```python
from build123d import *

# Parameters (mm, degrees)
SKETCH_1_R      = 1.5
EXTRUDE_1_DEPTH = 1.5
EXTRUDE_2_DEPTH = 15.5
SKETCH_3_W      = 49
SKETCH_3_H      = 51
EXTRUDE_3_DEPTH = 9.5
SKETCH_4_W      = 15
SKETCH_4_H      = 21
EXTRUDE_4_DEPTH = 13.5


with BuildPart() as part:
    # Эскиз1 → Бобышка-Вытянуть1 (new body)
    with BuildSketch(Plane(origin=(0, 0, 0), x_dir=(1, 0, 0), z_dir=(0, 1, 0))):
        with BuildLine():
            Line((3.5, 0), (52.5, 0))
            ThreePointArc((52.5, 0), (54.974873734, 1.025126266), (56, 3.5))
            Line((56, 3.5), (56, 83.5))
            ThreePointArc((56, 83.5), (54.974873734, 85.974873734), (52.5, 87))
            Line((52.5, 87), (3.5, 87))
            ThreePointArc((3.5, 87), (1.025126266, 85.974873734), (0, 83.5))
            Line((0, 83.5), (0, 3.5))
            ThreePointArc((0, 3.5), (1.025126266, 1.025126266), (3.5, 0))
        make_face()
        with Locations(Location((3.5, 83.5, 0), (0, 0, 270))):
            Circle(SKETCH_1_R, mode=Mode.SUBTRACT)
        with Locations(Location((52.5, 83.5, 0), (0, 0, 270))):
            Circle(SKETCH_1_R, mode=Mode.SUBTRACT)
        with Locations(Location((52.5, 25.5, 0), (0, 0, 270))):
            Circle(SKETCH_1_R, mode=Mode.SUBTRACT)
        with Locations(Location((3.5, 25.5, 0), (0, 0, 270))):
            Circle(SKETCH_1_R, mode=Mode.SUBTRACT)
    extrude(amount=EXTRUDE_1_DEPTH)

    # Эскиз2 → Бобышка-Вытянуть2 (add)
    with BuildSketch(Plane(origin=(0, 1.5, 0), x_dir=(1, 0, 0), z_dir=(0, 1, 0))):
        Polygon((20.5, 0), (28, 0), (36.5, 0), (36.5, 21), (20.5, 21), align=None)
        with BuildLine():
            Line((38.5, 21), (38.5, 0))
            Line((38.5, 0), (52.5, 0))
            ThreePointArc((52.5, 0), (53.005293538, 0.036666571), (53.5, 0.145898034))
            Line((53.5, 0.145898034), (53.5, 21))
            Line((53.5, 21), (38.5, 21))
        make_face()
    extrude(amount=EXTRUDE_2_DEPTH)

    # Эскиз3 → Бобышка-Вытянуть3 (add)
    with BuildSketch(Plane(origin=(0, 1.5, 0), x_dir=(1, 0, 0), z_dir=(0, 1, 0))):
        with Locations((28, 54.5)):
            Rectangle(SKETCH_3_W, SKETCH_3_H)
    extrude(amount=EXTRUDE_3_DEPTH)

    # Эскиз4 → Бобышка-Вытянуть4 (add)
    with BuildSketch(Plane(origin=(0, 1.5, 0), x_dir=(1, 0, 0), z_dir=(0, 1, 0))):
        with Locations((11, 10.5)):
            Rectangle(SKETCH_4_W, SKETCH_4_H)
    extrude(amount=EXTRUDE_4_DEPTH)


solid = part.part
```
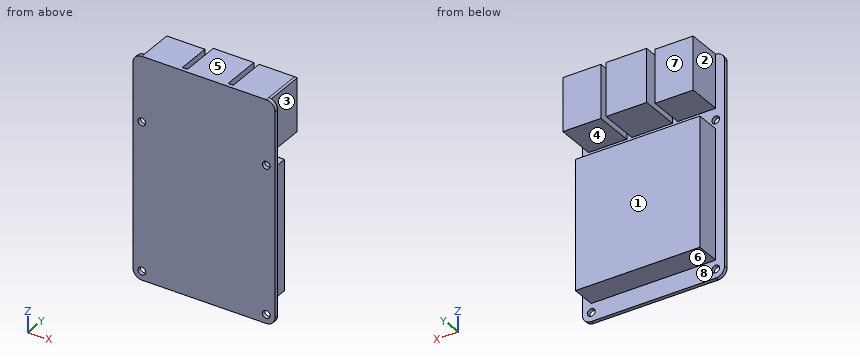
Can you work these out from the model? Positions are in its coordinate system, mm. Face numbers are marked on the shaded views. A direction names the side the tool comes from. Round coordinates to 2 decimals unless told otherwise and drop trailing zeros. Order: outer loops, then holes, each group sorted by start corner. A loop starts at its lowest first (then second) coordinate and runs counter-clockwise, first axis right, second up. Notation, with made-up numbers: (-21, 55.25) -> (1, 55.25) arc R34 cw to (1, 93.25) -> close; hole circle Ø7 at (7, 77). An arc over 180 degrees is marked (long way). Return JSON: item names as keys, results as strings. Group by question number.
1. If we section it at C-C, the plane z = -10: Write out the boundary of the cut face in (x, y), then the cut area to 3 significant figures.
2. I need wall thicknesses on line 1 (X direction, y = 0.55, z = -25.5); line 2 (X direction, y = 4, z = -16); line 3 (Z direction, x = 16, y = 9.5). Which ranges of each line are inside material? Lowest first, please. Write a range as [from, to].
3. We'd pull the mould along Z, two halves only. Please class the marked faces 6, 7 and 8: released by +Z, released by -Z, zero draft, split by the parting line, or undercut.
4. If we section it at B-B, the plane y = 9.75: Write out the boundary of the cut face in (x, z), then the cut area to 3 significant figures.
5. Will these pins go through, and if not, where does the flat tip stop? pin 1 (7 mm diameter, centred on x = 8.5, y = 5.5, fed in from -Z); pin 2 (7 mm diameter, centred on y = 11.5, z = -15.5, fed in from -X); pin 3 (1.5 mm diameter, centred on x = 21, z = -37.5, fed in from +Y); pin 4 (2.5 mm diameter, centred on x = 3.5, z = -25.5, fed in from +Y).
6. If we section it at D-D, the plane x = 9: Write out the boundary of the cut face in (y, z).
7. If we section it at A-A, the plane z = -25.5: Write out the boundary of the cut face in (x, y), then the cut area to 3 significant figures.
8. Which directions (+Z, -Z, +X, -X, +Y, -Y) give clear straight access to the entire face, cutting with the end or side of a thin tool? Please do the marked faces 1, 2, 3, 4 and 5.
Output values:
{
 "1": {"outline": "(0, 0) -> (56, 0) -> (56, 1.5) -> (53.5, 1.5) -> (53.5, 17) -> (38.5, 17) -> (38.5, 1.5) -> (36.5, 1.5) -> (36.5, 17) -> (20.5, 17) -> (20.5, 1.5) -> (18.5, 1.5) -> (18.5, 15) -> (3.5, 15) -> (3.5, 1.5) -> (0, 1.5) -> close", "area": "767 mm²"},
 "2": {"line 1": "[0, 2], [5, 51], [54, 56]", "line 2": "[3.5, 18.5], [20.5, 36.5], [38.5, 53.5]", "line 3": "[-80, -29], [-21, 0]"},
 "3": {"face 6": "released by -Z", "face 7": "zero draft", "face 8": "undercut"},
 "4": {"outline": "(3.5, -80) -> (52.5, -80) -> (52.5, -29) -> (3.5, -29) -> close; (3.5, -21) -> (18.5, -21) -> (18.5, 0) -> (3.5, 0) -> close; (20.5, -21) -> (36.5, -21) -> (36.5, 0) -> (20.5, 0) -> close; (38.5, -21) -> (53.5, -21) -> (53.5, -0.15) arc R3.5 ccw to (52.5, 0) -> (38.5, 0) -> close", "area": "3,460 mm²"},
 "5": {"pin 1": "z = -80", "pin 2": "x = 3.5", "pin 3": "y = 11", "pin 4": "through"},
 "6": {"outline": "(0, -87) -> (1.5, -87) -> (1.5, -80) -> (11, -80) -> (11, -29) -> (1.5, -29) -> (1.5, -21) -> (15, -21) -> (15, 0) -> (0, 0) -> close"},
 "7": {"outline": "(0, 0) -> (2, 0) -> (2, 1.5) -> (0, 1.5) -> close; (5, 0) -> (51, 0) -> (51, 1.5) -> (5, 1.5) -> close; (54, 0) -> (56, 0) -> (56, 1.5) -> (54, 1.5) -> close", "area": "75.0 mm²"},
 "8": {"face 1": "-Z, +X, -X, +Y", "face 2": "+Z, -Z, -X, +Y", "face 3": "+Z, -Z, +X, +Y", "face 4": "+X, -X, +Y", "face 5": "+Z, +X, -X, +Y, -Y"}
}
